The drawing under review shows one solid part. Ordinate dimensions are in mm from its lowest x, y, z. A direction names the side the tool comes from. Round coordinates to 2 decimals unless told otherwise and drop trailing zeros. Write each loop counter-clockwise with the first axis right and the second up, starting at its lowest first coordinate (ties: lowest second). Pieces come first, ordered by that corner, then holes.
Item 1: Add section B-B (z = 0.4). Give the boundary of the cut face in (x, y), plus the area to 3 significant figures.
Item 2: Clearance check with flat-ended pins moving along their axes: pin 1 Ø1 at (x, z) = (5, 1) entering from +Y; pin 2 Ø0.7 at (x, z) = (6, 0.5) entering from +Y; pin 3 Ø1.8 at (x, y) = (3.9, 3.9) entering from -Z; pin 4 Ø0.7 at (x, z) = (1.5, 0.5) entering from -Y. State where each tip first meets the part, or that it passes through.
Item 3: Add section C-C (z = 1.2). Give the boundary of the cut face in (x, y), plus the area to 3 significant figures.
Item 4: To check wall thickness, follow L1, parallel to X at y = 3.9, z = 2.85; L2, parallel to Y at x = 3.9, z = 0.3. State the ranges of each line that lie inside material, in increasing order.
Item 5: Draft analysis for pull direction X (two halves, no side actions). For the marked faces 3, 4 and 5, state which applies: +X half, -X half, draft (parallel to the pull), parting line (faces both ways), or undercut.
Item 6: Machinability: for the marked faces 1 and 2, which of the approach directions +Z, -Z, +X, -X, +Y, -Y give a long, thin tool a straight path to every point of the face, cutting with its end or side? Answer none if there is none.
Item 7: Add section A-A (x = 3.9). Give the boundary of the cut face in (y, z), plus the area to 3 significant figures.
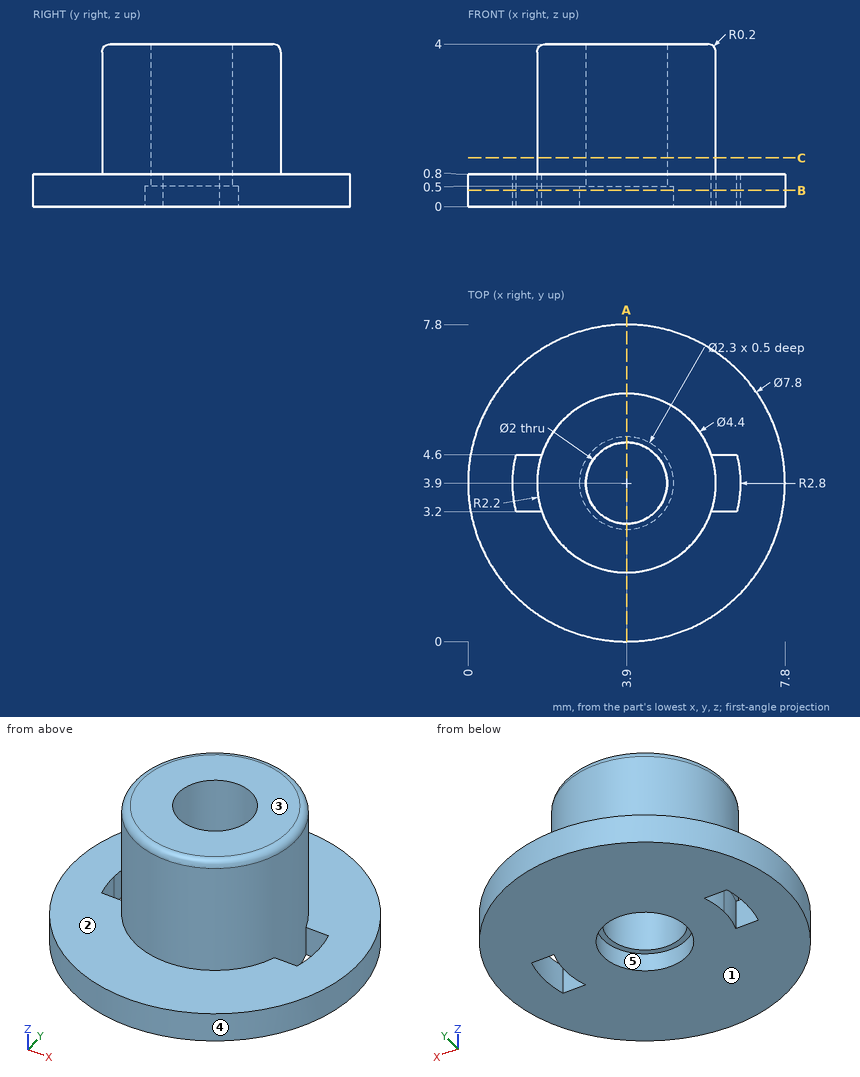
Numbers:
1. outline: circle Ø7.8 at (3.9, 3.9); hole (1.19, 3.2) - (1.81, 3.2) arc R2.2 cw to (1.81, 4.6) - (1.19, 4.6) arc R2.8 ccw to start; hole circle Ø2.3 at (3.9, 3.9); hole (5.99, 3.2) - (6.61, 3.2) arc R2.8 ccw to (6.61, 4.6) - (5.99, 4.6) arc R2.2 cw to start
1. area: 41.9 mm2
2. pin 1: stops at y = 7.75
2. pin 2: stops at y = 7.39
2. pin 3: passes through
2. pin 4: stops at y = 0.58
3. outline: circle Ø4.4 at (3.9, 3.9); hole circle Ø2 at (3.9, 3.9)
3. area: 12.1 mm2
4. L1: x = 1.7 to 2.9, 4.9 to 6.1
4. L2: y = 0 to 2.75, 5.05 to 7.8
5. face 3: draft
5. face 4: parting line
5. face 5: undercut
6. face 1: -Z, +X, -X, +Y, -Y
6. face 2: +Z
7. outline: (0, 0) - (2.75, 0) - (2.75, 0.5) - (2.9, 0.5) - (2.9, 4) - (1.9, 4) arc R0.2 ccw to (1.7, 3.8) - (1.7, 0.8) - (0, 0.8) - close; (4.9, 0.5) - (5.05, 0.5) - (5.05, 0) - (7.8, 0) - (7.8, 0.8) - (6.1, 0.8) - (6.1, 3.8) arc R0.2 ccw to (5.9, 4) - (4.9, 4) - close
7. area: 12.2 mm2
